Work out the finished part from the listing and answer in its coordinate system (mm). Face numbers are marked on the shaded views. Round coordinates to 2 decimals unless told otherwise and drop trailing zeros. Write each loop counter-clockwise with the first axis right and the second up, starting at its lowest first coordinate (ties: lowest second). Pieces come first, ordered by that corner, then holes. Notation, with made-up numbers: (33.5, 6.25) - (60.5, 6.25) arc R20 ccw to (60.5, 20.25) - close; hole circle Ø4 at (24.25, 72.5). An arc over 180 degrees is marked (long way). Answer as a JSON object with one key per item and string values.
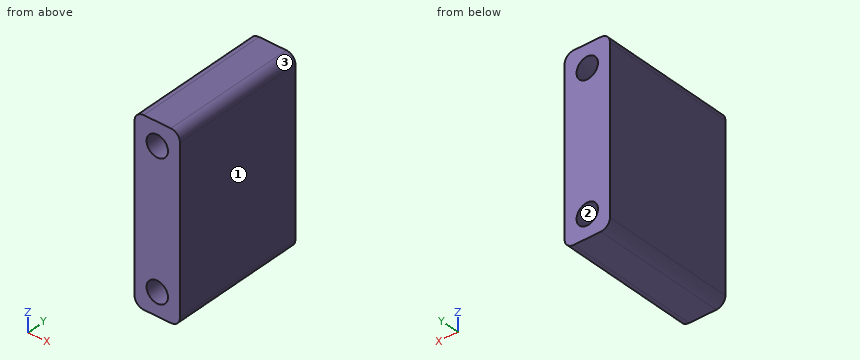
```python
from build123d import *

# Parameters (mm, degrees)
SKETCH2_R           = 2.05
BOSS_EXTRUDE1_DEPTH = 38.1
SKETCH3_R           = 3
CUT_EXTRUDE1_DEPTH  = 50


with BuildPart() as part:
    # Sketch2 → Boss-Extrude1 (new body)
    with BuildSketch(Plane(origin=(0, 0, 0), x_dir=(1, 0, 0), z_dir=(0, 1, 0))):
        with BuildLine():
            ThreePointArc((-25.4, -22.86), (-24.656051224, -24.656051224), (-22.86, -25.4))
            Line((-22.86, -25.4), (-15.24, -25.4))
            ThreePointArc((-15.24, -25.4), (-13.443948776, -24.656051224), (-12.7, -22.86))
            Line((-12.7, -22.86), (-12.7, 22.86))
            ThreePointArc((-12.7, 22.86), (-13.443948776, 24.656051224), (-15.24, 25.4))
            Line((-15.24, 25.4), (-19.05, 25.4))
            Line((-19.05, 25.4), (-22.86, 25.4))
            ThreePointArc((-22.86, 25.4), (-24.656051224, 24.656051224), (-25.4, 22.86))
            Line((-25.4, 22.86), (-25.4, 19.05))
            Line((-25.4, 19.05), (-25.4, -22.86))
        make_face()
        with Locations(Location((-19.05, -19.05, 0), (0, 0, 90))):
            Circle(SKETCH2_R, mode=Mode.SUBTRACT)
        with Locations(Location((-19.05, 19.05, 0), (0, 0, 90))):
            Circle(SKETCH2_R, mode=Mode.SUBTRACT)
    extrude(amount=BOSS_EXTRUDE1_DEPTH)

    # Sketch3 → Cut-Extrude1 (cut)
    with BuildSketch(Plane(origin=(0, 38.1, 0), x_dir=(1, 0, 0), z_dir=(0, 1, 0))):
        with Locations(Location((-19.05, 19.05, 0), (0, 0, 270))):
            Circle(SKETCH3_R)
        with Locations(Location((-19.05, -19.05, 0), (0, 0, 270))):
            Circle(SKETCH3_R)
    extrude(amount=-CUT_EXTRUDE1_DEPTH, mode=Mode.SUBTRACT)


solid = part.part
```
Item 1: Determine the mould class of the marked faces 1, 2 and 3 for opening direction Z: pulls with the +Z half, pulls with the -Z half, needs draft (parallel to the pull), parting line crosses it, or undercut.
Results found:
{"face 1": "needs draft", "face 2": "undercut", "face 3": "pulls with the +Z half"}
Item 2: This flat-tipped pin is pushed along its axis until it touches: P1, Ø3.5, axis at x = -19.05, z = -19.05, coming from the -Y side. Where does it stop, or does it pass through?
Results found:
{"P1": "through"}
Item 3: A cutting plane is placed at C-C (z = -19.05). Write down the section's boundary in (x, y).
Results found:
{"outline": "(-25.4, 0) - (-22.05, 0) - (-22.05, 38.1) - (-25.4, 38.1) - close; (-16.05, 0) - (-12.7, 0) - (-12.7, 38.1) - (-16.05, 38.1) - close"}
Item 4: A cutting plane is placed at A-A (x = -19.05). Write down the section's boundary in (y, z), and give its area (3 significant figures).
Results found:
{"outline": "(0, -25.4) - (38.1, -25.4) - (38.1, -22.05) - (0, -22.05) - close; (0, -16.05) - (38.1, -16.05) - (38.1, 16.05) - (0, 16.05) - close; (0, 22.05) - (38.1, 22.05) - (38.1, 25.4) - (0, 25.4) - close", "area": "1,480 mm²"}
Item 5: A cutting plane is placed at D-D (x = -16.75). Write down the section's boundary in (y, z), and give its area (3 significant figures).
Results found:
{"outline": "(0, -25.4) - (38.1, -25.4) - (38.1, -20.98) - (0, -20.98) - close; (0, -17.12) - (38.1, -17.12) - (38.1, 17.12) - (0, 17.12) - close; (0, 20.98) - (38.1, 20.98) - (38.1, 25.4) - (0, 25.4) - close", "area": "1,640 mm²"}
Item 6: A cutting plane is placed at B-B (y = 7.5). Write down the section's boundary in (x, z).
Results found:
{"outline": "(-25.4, -22.86) arc R2.54 ccw to (-22.86, -25.4) - (-15.24, -25.4) arc R2.54 ccw to (-12.7, -22.86) - (-12.7, 22.86) arc R2.54 ccw to (-15.24, 25.4) - (-22.86, 25.4) arc R2.54 ccw to (-25.4, 22.86) - close; hole circle Ø6 at (-19.05, -19.05); hole circle Ø6 at (-19.05, 19.05)"}
Item 7: Consider line 1 along X through (y, z) = (12, 19.05); line 2 along Z through (x, y) = (-16.5, 7); line 3 along Z through (x, y) = (-18.25, 11.5). Determine where each line is inside the solid, lowest interval first.
Results found:
{"line 1": "-25.4 to -22.05, -16.05 to -12.7", "line 2": "-25.4 to -20.63, -17.47 to 17.47, 20.63 to 25.4", "line 3": "-25.4 to -21.94, -16.16 to 16.16, 21.94 to 25.4"}
